Can you work these out from the model? Positions are in its coordinate system, mm. A direction names the side the tool comes from. Give positions to 0.01 mm unless a question says otherwise; leave off trailing zeros. Loops run counter-clockwise (first coordinate to the right, second up) from the corner with the lowest first, then second, coordinate; pieces in that order, holes last. Notation, with made-up numbers: (-22.75, 88.5) - (26.25, 88.5) arc R25 cw to (26.25, 117.5) - close; hole circle Ø6 at (46.25, 44). An arc over 180 degrees is marked (long way). Answer as a JSON object with one key per item and string values.
```python
from build123d import *

# Parameters (mm, degrees)
F1_DEPTH  = 48
F2_R      = 10
F3_R      = 10
F5_D      = 13
F8_DEPTH  = 25
F6_R      = 2.5
F9_DEPTH  = 25
F10_R     = 2.5883727543
F11_DEPTH = 35


with BuildPart() as f1:
    # F0 (on Right) → F1 (new body)
    with BuildSketch(Plane.YZ):
        with BuildLine():
            ThreePointArc((27.9105714739, 11), (29.4730143031, 5.5983415304), (30, 0))
            Line((30, 0), (57, 0))
            Line((57, 0), (57, 41))
            Line((57, 41), (46, 41))
            Line((46, 41), (46, 10.8391446993))
            Line((46, 10.8391446993), (27.9105714739, 11))
        make_face()
        with BuildLine():
            Line((-50, 0), (-30, 0))
            ThreePointArc((-30, 0), (-29.4730143031, 5.5983415304), (-27.9105714739, 11))
            Line((-27.9105714739, 11), (-50, 11))
            Line((-50, 11), (-50, 0))
        make_face()
        with BuildLine():
            ThreePointArc((-19, 0), (0, 19), (19, 0))
            Line((19, 0), (30, 0))
            ThreePointArc((30, 0), (29.4730143031, 5.5983415304), (27.9105714739, 11))
            ThreePointArc((27.9105714739, 11), (0, 30), (-27.9105714739, 11))
            ThreePointArc((-27.9105714739, 11), (-29.4730143031, 5.5983415304), (-30, 0))
            Line((-30, 0), (-19, 0))
        make_face()
    extrude(amount=F1_DEPTH)

    # F2
    f2_edges = [f1.edges().sort_by_distance(p)[0] for p in [
        (0, -50, 5.5),
    ]]
    fillet(f2_edges, radius=F2_R)

    # F3
    f3_edges = [f1.edges().sort_by_distance(p)[0] for p in [
        (48, -50, 5.5),
        (48, 51.5, 41),
        (0, 51.5, 41),
        (24, 57, 0),
    ]]
    fillet(f3_edges, radius=F3_R)

    # F5 (through all)
    with Locations(Plane.XY.offset(11)):
        with Locations((38, -40), (10, -40)):
            Hole(F5_D / 2)

    # F7 (on face) → F8 (cut)
    with BuildSketch(Plane(origin=(0, 57, 0), x_dir=(-1, 0, 0), z_dir=(0, 1, 0))):
        with BuildLine():
            Line((-31.0717061657, 41), (-31.0717061657, 24.151092889))
            ThreePointArc((-31.0717061657, 24.151092889), (-24.4338531361, 17.6483010112), (-18.0777366792, 24.4267358331))
            Line((-18.0777366792, 24.4267358331), (-18.0777366792, 41))
            Line((-18.0777366792, 41), (-31.0717061657, 41))
        make_face()
    extrude(amount=-F8_DEPTH, mode=Mode.SUBTRACT)

    # F6 (on Top) → F9 (cut)
    with BuildSketch(Plane.XY):
        with Locations((23.1874617344, 0)):
            Circle(F6_R)
    extrude(amount=-F9_DEPTH, mode=Mode.SUBTRACT)

    # F10 (on Top) → F11 (cut)
    with BuildSketch(Plane.XY):
        with Locations((24.0040104836, 0)):
            Circle(F10_R)
    extrude(amount=F11_DEPTH, mode=Mode.SUBTRACT)


solid = f1.part
```
1) I'm going to push flat-ended pins straight in: P1, Ø8, axis at x = 41, y = 4, coming from the +Z side; P2, Ø1.5, axis at x = 21, y = 0.5, coming from the -Z side; P3, Ø10, axis at x = 16.5, y = 12.5, coming from the -Z side. Where does each tip first touch, or does it pass through?
Check sheet entries:
{"P1": "z = 30", "P2": "z = 18.96", "P3": "z = 7.4"}
2) Imagine slicing it at B-B on y = 0. Write out the boundary of the cut face in (x, z), and give its area (3 significant figures).
Check sheet entries:
{"outline": "(0, 19) - (21.42, 19) - (21.42, 30) - (0, 30) - close; (26.59, 19) - (48, 19) - (48, 30) - (26.59, 30) - close", "area": "471 mm2"}
3) If we mould it in two halves opening along X, with no side actions, what happens to faces 4 (the flat face through (0, 19, 16)), 5 (the cylindrical face through (22.096, 1.749, 24.333)), 6 (the cylindrical face through (44.99, -47.15, 5.42)), 7 (the flat face through (18.078, 52, 33))? For each: released by +X, released by -X, zero draft, split by the parting line, or undercut.
Check sheet entries:
{"face 4": "released by -X", "face 5": "undercut", "face 6": "released by +X", "face 7": "undercut"}
4) I need wall thicknesses on L1, parallel to Y at x = 40, z = 5.5; L2, parallel to Y at x = 38, z = 5; L3, parallel to Z at x = 6.5, y = 29. Which ranges of each line are inside material? Lowest first, please.
Check sheet entries:
{"L1": "-49.8 to -46.18, -33.82 to -18.19, 18.19 to 55.93", "L2": "-50 to -46.5, -33.5 to -18.33, 18.33 to 55.66", "L3": "0 to 10.99"}
5) Imagine slicing it at D-D on z = 29. Write out the boundary of the cut face in (x, y).
Check sheet entries:
{"outline": "(0, -7.68) - (48, -7.68) - (48, 7.68) - (0, 7.68) - close; (0, 46) - (18.08, 46) - (18.08, 57) - (0, 57) - close; (31.07, 46) - (48, 46) - (48, 57) - (31.07, 57) - close; hole circle Ø5.18 at (24, 0)"}
6) Which directions (+Z, -Z, +X, -X, +Y, -Y) give clear straight access to the entire face, cutting with the end or side of a thin tool? Please do faces 1 (the flat face through (24, -39, 11)), 2 (the flat face through (31.072, 52, 33)), 3 (the flat face through (18, 46, 19)).
Check sheet entries:
{"face 1": "+Z, +X, -X, -Y", "face 2": "+Z, +Y", "face 3": "+Z, +X, -X"}
7) Imagine slicing it at A-A on z = 37. Write out the boundary of the cut face in (x, y), and give its area (3 significant figures).
Check sheet entries:
{"outline": "(2, 46) - (18.08, 46) - (18.08, 57) - (2, 57) - close; (31.07, 46) - (46, 46) - (46, 57) - (31.07, 57) - close", "area": "341 mm2"}
8) Imagine slicing it at C-C on x = 42.5. Write out the boundary of the cut face in (y, z).
Check sheet entries:
{"outline": "(-48.93, 0) - (-44.69, 0) - (-44.69, 11) - (-48.93, 11) - close; (-35.31, 0) - (-19, 0) arc R19 cw to (19, 0) - (47, 0) arc R10 ccw to (57, 10) - (57, 39.93) - (46, 39.93) - (46, 10.84) - (27.91, 11) arc R30 ccw to (-27.91, 11) - (-35.31, 11) - close"}
